Source: CAD feature listing. Evaluate the final solid. Frame: model axes, mm. A direction names the side the tool comes from. Round coordinates to 2 decimals unless told otherwise and drop trailing zeros. Order: outer loops, then holes, each group sorted by start corner. A loop starts at its lowest first (then second) coordinate and runs counter-clockwise, first axis right, second up. Notation, with made-up numbers: (64.25, -4.75) - (90.25, -4.75) arc R25 ccw to (90.25, 25.25) - close; hole circle Ø7 at (60, -12). An arc over 180 degrees is marked (long way). Put each result on its own line as item: value. Start each with the question number.
1) Access query for faces 1 (the face through (-1, 0, -76)), 2 (the face through (-31.172, 46.056, -138.923)). Directions: +Z, -Z, +X, -X, +Y, -Y. A direction counts if a zero-diameter tool reaches every point of the face in a straight line with its end or side. Return the directions, or none.
2) Section A-A on z = -130. Output: boundary loops of the cut face in (x, y).
3) Section C-C on y = 18.5. Output: boundary loops of the cut face in (x, z), then the cut area to 3 significant figures.
4) Mould query, pull axis Z, two halves, no side actions, for faces 3 (the face through (-24, 42, -18)), 4 (the face through (-1, 25, 0)), 5 (the face through (50, 24.7, -74)). Classes: +Z half, -Z half, draft (parallel to the pull), parting line (faces both ways), or undercut.
5) Contact query for a flat-ended pin moving along its axis: P1, Ø9, axis at x = 30, z = -24, coming from the +Y side. Output: stop coordinate, or through.
6) Section B-B on y = 29. Output: boundary loops of the cut face in (x, z).
7) Section D-D on x = 30. Output: boundary loops of the cut face in (y, z).
8) Line query: probe 1 along X at (y, z) = (20.5, -130); probe 2 along Z at (x, y) = (30, 11); probe 3 along X at (y, z) = (48, -130). Output: solid intervals per line, ascending. Write a range as [from, to].
Autodesk Inventor part; units mm, degrees
ref_plane "YZ Plane" through (0, 0, 0) normal (1, 0, 0) x (0, 1, 0)
ref_plane "XZ Plane" through (0, 0, 0) normal (0, 1, 0) x (-1, 0, 0)
ref_plane "XY Plane" through (0, 0, 0) normal (0, 0, 1) x (1, 0, 0)
sketch "Sketch1" plane through (0, 0, 0) normal (1, 0, 0) x (0, 1, 0)
  line L0 (0, 0) -> (50, 0)
  line L1 (50, -150) -> (0, -150)
  line L2 (0, -150) -> (0, 0)
  arc A0 (50, -50) -> (50, -100) centre (50, -75) ccw
  line L3 (50, 0) -> (50, -50)
  line L4 (50, -100) -> (50, -150)
  dimension "d0" = 150
  dimension "d2" = 50
  dimension "d3" = 50
extrude "Extrusion1" add sketch "Sketch1" along normal mid plane 100
sketch "Sketch2" plane through (-50, 50, 0) normal (0, 1, 0) x (1, 0, 0)
  circle A0 centre (20, 20) radius 6
  circle A1 centre (20, 20) radius 9
  line L0 (0, 0) -> (100, 0)
  line L1 (0, 0) -> (0, 50)
  point P0 (50, 0)
  dimension "d6" = 18
  dimension "d7" = 12
  dimension "d8" = 20
  dimension "d9" = 20
extrude "Extrusion2" cut sketch "Sketch2" against normal through all contours A0
extrude "Extrusion3" cut sketch "Sketch2" against normal blind 8 contours A0 | A1
pattern_linear "Rectangular Pattern1" count 2 spacing 110 along (0, 0, -1) count 2 spacing 60 along (1, 0, 0) of "Extrusion3", "Extrusion2"
properties part number "Partdia16"
Answer sheet:
1. face 1: +Z, -Z, +X, -X, -Y
1. face 2: +Y
2. outline: (-50, 0) - (-36, 0) - (-36, 42) - (-39, 42) - (-39, 50) - (-50, 50) - close; (-24, 0) - (24, 0) - (24, 42) - (21, 42) - (21, 50) - (-21, 50) - (-21, 42) - (-24, 42) - close; (36, 0) - (50, 0) - (50, 50) - (39, 50) - (39, 42) - (36, 42) - close
3. outline: (-50, -150) - (50, -150) - (50, 0) - (-50, 0) - close; hole circle Ø12 at (-30, -130); hole circle Ø12 at (-30, -20); hole circle Ø12 at (30, -130); hole circle Ø12 at (30, -20)
3. area: 14,500 mm^2
4. face 3: undercut
4. face 4: +Z half
4. face 5: draft
5. P1: y = 42
6. outline: (-50, -150) - (50, -150) - (50, -88.56) - (-50, -88.56) - close; (-50, -61.44) - (50, -61.44) - (50, 0) - (-50, 0) - close; hole circle Ø12 at (-30, -130); hole circle Ø12 at (-30, -20); hole circle Ø12 at (30, -130); hole circle Ø12 at (30, -20)
7. outline: (0, -150) - (50, -150) - (50, -139) - (42, -139) - (42, -136) - (0, -136) - close; (0, -124) - (42, -124) - (42, -121) - (50, -121) - (50, -100) arc R25 cw to (50, -50) - (50, -29) - (42, -29) - (42, -26) - (0, -26) - close; (0, -14) - (42, -14) - (42, -11) - (50, -11) - (50, 0) - (0, 0) - close
8. probe 1: [-50, -36], [-24, 24], [36, 50]
8. probe 2: [-150, -136], [-124, -26], [-14, 0]
8. probe 3: [-50, -39], [-21, 21], [39, 50]
